from build123d import *

# Parameters (mm, degrees)
F_1_4_0_24_DIAMETER_HOLE1_D = 6.096


with BuildPart() as part:
    # Sketch1 → Revolve1 (revolve)
    with BuildSketch(Plane.XY):
        Polygon((0, 0), (0, 3.937), (0.635, 3.937), (1.5494, 4.8514), (1.5494, 5.334), (2.921, 5.334), (2.921, 3.937), (9.525, 3.937), (9.525, 0), align=None)
    revolve(axis=Axis((-1.987928477, 0, 0), (1, 0, 0)))

    # 1/4 (0.24) Diameter Hole1 (through all)
    with Locations(Plane(origin=(9.525, 0, 0), x_dir=(0, 0, -1), z_dir=(1, 0, 0))):
        with Locations((0, 0)):
            Hole(F_1_4_0_24_DIAMETER_HOLE1_D / 2)


solid = part.part
Model file for the job. Use its own axes, mm. A direction names the side the tool comes from. Round coordinates to 2 decimals unless told otherwise and drop trailing zeros. Order: outer loops, then holes, each group sorted by start corner. A loop starts at its lowest first (then second) coordinate and runs counter-clockwise, first axis right, second up.
(1) Drill centre lines: line 1 (Y direction, x = 1.75, z = -1); line 2 (Y direction, x = 4.5, z = -0.75); line 3 (Z direction, x = 4.5, y = 2.25). Where is each one in solid material? Low to high.
(2) Band-saw the part on C-C (x = 7.5). List the corners of the cut face in (y, z).
(3) Band-saw the part on A-A (z = 0). List the corners of the cut face in (x, y) (3 decimals), then the cut area to 3 significant figures.
(4) 3-axis set-ups, long thin cutter, end or side, ignore diameter. For faces 1 (the face through (6.269, -0.853, -3.843)), 2 (the face through (1.549, -1, -5)), 3 (the face through (4.7, 3.02, -0.4)): which of +Z, -Z, +X, -X, +Y, -Y reach the whole face in a straight line?
(5) Pin check, flat tips, straight feed: pin 1 (2 mm diameter, centred on x = 8.5, y = -4, fed in from +Z); pin 2 (1.5 mm diameter, centred on x = 7.5, z = 3, fed in from -Y); pin 3 (1 mm diameter, centred on x = 6.5, y = 0.5, fed in from -Z). Stop position of each tip, or through.
Verdict:
1. line 1: y = -5.24 to -2.88, 2.88 to 5.24
1. line 2: y = -3.86 to -2.95, 2.95 to 3.86
1. line 3: z = -3.23 to -2.06, 2.06 to 3.23
2. outline: circle Ø7.87 at (0, 0); hole circle Ø6.1 at (0, 0)
3. outline: (0, -3.937) - (0.635, -3.937) - (1.549, -4.851) - (1.549, -5.334) - (2.921, -5.334) - (2.921, -3.937) - (9.525, -3.937) - (9.525, -3.048) - (0, -3.048) - close; (0, 3.048) - (9.525, 3.048) - (9.525, 3.937) - (2.921, 3.937) - (2.921, 5.334) - (1.549, 5.334) - (1.549, 4.851) - (0.635, 3.937) - (0, 3.937) - close
3. area: 21.6 mm2
4. face 1: +X
4. face 2: -X
4. face 3: +X, -X
5. pin 1: stops at z = 2.55
5. pin 2: stops at y = -3.23
5. pin 3: stops at z = -3.94
